from build123d import *

# Parameters (mm, degrees)
SKETCH1_W           = 23
SKETCH1_H           = 3
SKETCH1_W_2         = 3
SKETCH1_H_2         = 29
BOSS_EXTRUDE1_DEPTH = 16
HOLE1_AT_2_COUNT    = 2
HOLE1_AT_2_PITCH    = 10
SKETCH5_R           = 6.25
CUT_EXTRUDE1_DEPTH  = 39.691084244


with BuildPart() as part:
    # Sketch1 → Boss-Extrude1 (new body)
    with BuildSketch(Plane(origin=(0, 0, 0), x_dir=(0, 0, -1), z_dir=(1, 0, 0))):
        with Locations((11.5, -1.5)):
            Rectangle(SKETCH1_W, SKETCH1_H)
        with Locations((21.5, 14.5)):
            Rectangle(SKETCH1_W_2, SKETCH1_H_2)
    extrude(amount=BOSS_EXTRUDE1_DEPTH)

    # Sketch4 → Hole1 (revolve, cut)
    with BuildSketch(Plane(origin=(8, 0, -5), x_dir=(0, 0, 1), z_dir=(1, 0, 0))):
        Polygon((0, 0), (0, 3), (1.6, 3), (1.6, 1.746093602), (3.2, 0), align=None)
    hole1 = revolve(axis=Axis((8, 6.445314094, -5), (0, -1, 0)), mode=Mode.SUBTRACT)

    # Hole1 at 2: Hole1 ×2
    with Locations(*[(0, 0, -i * HOLE1_AT_2_PITCH) for i in range(1, HOLE1_AT_2_COUNT)]):
        add(hole1, mode=Mode.SUBTRACT)

    # Sketch5 → Cut-Extrude1 (cut, through all)
    with BuildSketch(Plane.XY.offset(-20)):
        with Locations((8, 15.5)):
            Circle(SKETCH5_R)
    extrude(amount=-CUT_EXTRUDE1_DEPTH, mode=Mode.SUBTRACT)


solid = part.part
Could you check a few things on this model? Use its own coordinates, in mm. A direction names the side the tool comes from. Give positions to 0.01 mm unless a question says otherwise; leave off trailing zeros. Write each loop counter-clockwise with the first axis right and the second up, starting at its lowest first coordinate (ties: lowest second). Pieces come first, ordered by that corner, then holes. Notation, with made-up numbers: (30.5, 20.25) -> (40.5, 20.25) arc R11 cw to (40.5, 34.25) -> close; hole circle Ø1 at (29, 57). An arc over 180 degrees is marked (long way). Answer as CSV lines item,"result". Start each with the question number.
(1) If we section it at B-B, the plane y = 15.5: Write out the boundary of the cut face in (x, z).
(2) Please list where these lines run through material, in increasing order: line 1 (X direction, y = -2.15, z = -15); line 2 (Y direction, x = 8, z = -21.9); line 3 (Y direction, x = 13.25, z = -18).
(3) If we mould it in two halves opening along X, with no side actions, what happens to faces 3 (the face through (0, 7, -21)), 4 (the face through (8, -2, 0)), 5 (the face through (9.56, -2.36, -5.35))? For each: +X half, -X half, draft (parallel to the pull), parting line (faces both ways), or undercut.
(4) Which directions (+Z, -Z, +X, -X, +Y, -Y) give clear straight access to the entire face, cutting with the end or side of a thin tool? Please do faces 1 (the face through (8, 8, -20)), 2 (the face through (8, 9, -23)).
(5) If we section it at D-D, the plane x = 8: Write out the boundary of the cut face in (y, z), and give its area (3 significant figures).
(6) I'm going to push flat-ended pins straight in: pin 1 Ø8 at (x, z) = (4, -19) entering from +Y; pin 2 Ø1.5 at (x, z) = (13.5, -19) entering from +Y; pin 3 Ø8 at (x, y) = (8, 12) entering from +Z. Where does each tip first touch, or does it pass through?
(7) If we section it at A-A, the plane x = 4.25: Write out the boundary of the cut face in (y, z), and give its area (3 significant figures).
(8) If we section it at C-C, the plane z = -15: Write out the boundary of the cut face in (x, y), and give its area (3 significant figures).
Answer list:
1,outline,"(0, -23) -> (1.75, -23) -> (1.75, -20) -> (0, -20) -> close; (14.25, -23) -> (16, -23) -> (16, -20) -> (14.25, -20) -> close"
2,line 1,"0 to 6.4, 9.6 to 16"
2,line 2,"-3 to 9.25, 21.75 to 29"
2,line 3,"-3 to 0"
3,face 3,"-X half"
3,face 4,"draft"
3,face 5,"undercut"
4,face 1,"+Z, +X, -X, +Y"
4,face 2,"-Z, +X, -X, +Y, -Y"
5,outline,"(-3, -23) -> (9.25, -23) -> (9.25, -20) -> (0, -20) -> (0, -18.2) -> (-1.75, -16.6) -> (-3, -16.6) -> close; (-3, -13.4) -> (-1.75, -13.4) -> (0, -11.8) -> (0, -8.2) -> (-1.75, -6.6) -> (-3, -6.6) -> close; (-3, -3.4) -> (-1.75, -3.4) -> (0, -1.8) -> (0, 0) -> (-3, 0) -> close; (21.75, -23) -> (29, -23) -> (29, -20) -> (21.75, -20) -> close"
5,area,"93.7 mm^2"
6,pin 1,"y = 29"
6,pin 2,"y = 0"
6,pin 3,"z = -20"
7,outline,"(-3, -23) -> (10.5, -23) -> (10.5, -20) -> (0, -20) -> (0, 0) -> (-3, 0) -> close; (20.5, -23) -> (29, -23) -> (29, -20) -> (20.5, -20) -> close"
7,area,"126 mm^2"
8,outline,"(0, -3) -> (6.4, -3) -> (6.4, -1.75) -> (4.8, 0) -> (0, 0) -> close; (9.6, -3) -> (16, -3) -> (16, 0) -> (11.2, 0) -> (9.6, -1.75) -> close"
8,area,"35.6 mm^2"
